The model under review builds one solid part; all positions refer to its coordinate system, in mm. A direction names the side the tool comes from. Give positions to 0.01 mm unless a question says otherwise; leave off trailing zeros. Order: outer loops, then holes, each group sorted by start corner. A loop starts at its lowest first (then second) coordinate and runs counter-clockwise, first axis right, second up. Notation, with made-up numbers: (-33, 29) - (0, 29) arc R25 cw to (0, 52) - close; hole circle Ø6 at (44.25, -6). An arc over 180 degrees is marked (long way). Use CSV: the item, a comma, the result in double quotes. Start each with the question number.
1. To check wall thickness, follow line 1 (Z direction, x = 47.5, y = 25); line 2 (X direction, y = -28, z = 8.5); line 3 (Y direction, x = -2.5, z = 18). State the ranges of each line that lie inside material, in increasing order. Write a range as [from, to].
2. Take a section at A-A, the plane x = 0. State the section outline as (y, z) points, then the cut area to 3 significant figures.
3. Take a section at D-D, the plane z = 23.5. State the section outline as (x, y) points.
4. Take a section at C-C, the plane z = 5. State the section outline as (x, y) points, then the cut area to 3 significant figures.
5. Machinability: for faces 1 (the cylindrical face through (-10.316, -7.91, 34.79)), 2 (the flat face through (0, 0, 50)), which of the approach directions +Z, -Z, +X, -X, +Y, -Y give a long, thin tool a straight path to every point of the face, cutting with its end or side? Answer none if there is none.
6. Draft analysis for pull direction X (two halves, no side actions). For faces 3 (the cylindrical face through (69.15, 21.78, 3.45)), 4 (the flat face through (-1, 1, 0)), state which applies: released by +X, released by -X, zero draft, split by the parting line, or undercut.
7. For pin 1 (10 mm diameter, centred on x = -51, y = 15.5, fed in from +Z); pin 2 (2 mm diameter, centred on x = -8.5, z = 23, fed in from -Y), all flat-tipped, find the tip position at first contact; note any pin that passes through.
```python
from build123d import *

# Parameters (mm, degrees)
F0_R     = 72.5
F1_DEPTH = 10
F2_R     = 16
F3_DEPTH = 10
F4_R     = 13
F5_DEPTH = 30
F6_R     = 3
F7_R     = 5


with BuildPart() as f1:
    # F0 (on Top) → F1 (new body)
    with BuildSketch(Plane.XY):
        Circle(F0_R)
    extrude(amount=F1_DEPTH)

    # F2 (on face) → F3 (join)
    with BuildSketch(Plane.XY.offset(10)):
        Circle(F2_R)
    extrude(amount=F3_DEPTH)

    # F4 (on face) → F5 (join)
    with BuildSketch(Plane.XY.offset(20)):
        Circle(F4_R)
    extrude(amount=F5_DEPTH)

    # F6
    f6_edges = [f1.edges().sort_by_distance(p)[0] for p in [
        (-72.5, 0, 10),
    ]]
    fillet(f6_edges, radius=F6_R)

    # F7
    f7_edges = [f1.edges().sort_by_distance(p)[0] for p in [
        (-72.5, 0, 7),
        (-69.5, 0, 10),
        (-16, 0, 10),
    ]]
    fillet(f7_edges, radius=F7_R)


solid = f1.part
```
Determined:
1,line 1,"z = [0, 10]"
1,line 2,"x = [-66.44, 66.44]"
1,line 3,"y = [-15.8, 15.8]"
2,outline,"(-72.5, 0) - (72.5, 0) - (72.5, 7) arc R3 ccw to (69.5, 10) - (21, 10) arc R5 cw to (16, 15) - (16, 20) - (13, 20) - (13, 50) - (-13, 50) - (-13, 20) - (-16, 20) - (-16, 15) arc R5 cw to (-21, 10) - (-69.5, 10) arc R3 ccw to (-72.5, 7) - close"
2,area,"2,560 mm²"
3,outline,"circle Ø26 at (0, 0)"
4,outline,"circle Ø145 at (0, 0)"
4,area,"16,500 mm²"
5,face 1,"+Z"
5,face 2,"+Z, +X, -X, +Y, -Y"
6,face 3,"split by the parting line"
6,face 4,"zero draft"
7,pin 1,"stops at z = 10"
7,pin 2,"stops at y = -10.62"
